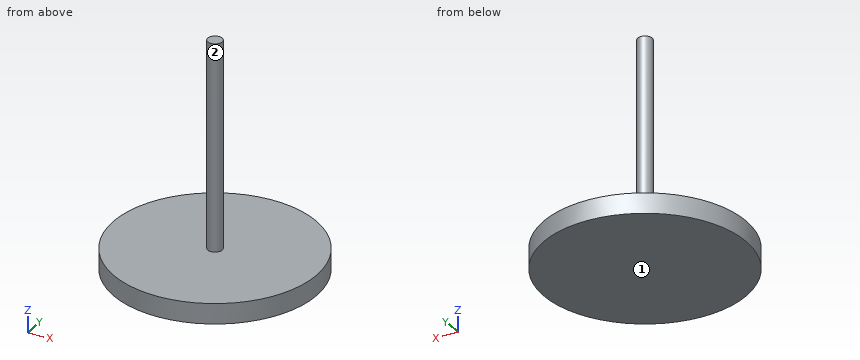
Solid Edge part; units mm, degrees
sketch "Sketch1" plane through (0, 0, 0) normal (0, 0, 1) x (1, 0, 0)
  circle A0 centre (0, 0) radius 8.89
  circle A1 centre (0, 0) radius 0.635
extrude "Protrusion1" add sketch "Sketch1" along normal mid plane 1.778
sketch "Sketch2" plane through (0, 0, 0) normal (0, 0, 1) x (1, 0, 0)
  circle A0 centre (0, 0) radius 0.635
extrude "Protrusion2" add sketch "Sketch2" along normal blind 18.9992
sketch "Sketch3" plane through (0, 0, 0) normal (0, 0, 1) x (1, 0, 0)
  circle A0 centre (0, 0) radius 0.635
extrude "Protrusion3" add sketch "Sketch3" along normal up to surface (0.889 mm away) from surface at -0.889
The listing builds one solid part. Answer for the finished solid, in the listing's coordinates (mm). Face numbers are marked on the shaded views. A direction names the side the tool comes from. Round coordinates to 2 decimals unless told otherwise and drop trailing zeros. Loops run counter-clockwise (first coordinate to the right, second up) from the corner with the lowest first, then second, coordinate; pieces in that order, holes last. Notation, with made-up numbers: (-11, -34.75) - (35, -34.75) arc R18 ccw to (35, -2.75) - close; hole circle Ø5 at (-2, 67). An arc over 180 degrees is marked (long way). Return JSON: item names as keys, results as strings. Group by question number.
1. Consider probe 1 along Z at (x, y) = (7, 1.75); probe 2 along X at (y, z) = (-0.5, 14.5); probe 3 along Y at (x, z) = (0.25, 7). Determine where each line is inside the solid, lowest interval first.
2. Which of the six approach directions +Z, -Z, +X, -X, +Y, -Y give full straight-line access (tool end or side, diameter ignored) to the marked faces 1 and 2?
3. Each of these flat-tipped pins is pushed along its axis until it touches: P1, Ø6, axis at y = -2.5, z = 5.5, coming from the -X side (3 decimals); P2, Ø2, axis at x = -1.5, y = -4.5, coming from the +Z side. Where does it stop, or does it pass through?
4. The part is cut by section C-C on z = 6.25. Determine the outline of the cut face in (x, y) (3 decimals), then the cut area to 3 significant figures.
5. The part is cut by section A-A on y = 0. Determine the outline of the cut face in (x, z) (3 decimals).
6. The part is cut by section D-D on x = 6.25. Determine the outline of the cut face in (y, z), then the cut area to 3 significant figures.
Resolved:
{
 "1": {"probe 1": "z = -0.89 to 0.89", "probe 2": "x = -0.39 to 0.39", "probe 3": "y = -0.58 to 0.58"},
 "2": {"face 1": "-Z, +X, -X, +Y, -Y", "face 2": "+Z"},
 "3": {"P1": "stops at x = -0.635", "P2": "stops at z = 0.89"},
 "4": {"outline": "circle Ø1.27 at (0, 0)", "area": "1.27 mm²"},
 "5": {"outline": "(-8.89, -0.889) - (8.89, -0.889) - (8.89, 0.889) - (0.635, 0.889) - (0.635, 18.999) - (-0.635, 18.999) - (-0.635, 0.889) - (-8.89, 0.889) - close"},
 "6": {"outline": "(-6.32, -0.89) - (6.32, -0.89) - (6.32, 0.89) - (-6.32, 0.89) - close", "area": "22.5 mm²"}
}
